Read the model definition and answer for the solid it produces. Units are mm, in the model's axes. Give positions to 0.01 mm unless a question says otherwise; leave off trailing zeros. Order: outer loops, then holes, each group sorted by start corner. A loop starts at its lowest first (then second) coordinate and runs counter-clockwise, first axis right, second up. Notation, with made-up numbers: M 80.25,30.25 L 109.25,30.25 A10 ccw 109.25,38.25 Z; hole C -29,9.5 d11. An arc over 180 degrees is marked long. Write item = value, one per line. Start each with the question number.
from build123d import *

# Parameters (mm, degrees)
SKETCH1_W                    = 25.4
SKETCH1_H                    = 25.4
SKETCH1_W_2                  = 22.225
SKETCH1_H_2                  = 22.225
EXTRUDE_THIN1_DEPTH          = 387.35
F_10_0_1935_DIAMETER_HOLE1_D = 4.9149
F_10_0_1935_DIAMETER_HOLE2_D = 4.9149


with BuildPart() as part:
    # Sketch1 → Extrude-Thin1 (new body)
    with BuildSketch(Plane(origin=(0, 0, 0), x_dir=(0, 0, -1), z_dir=(1, 0, 0))):
        Rectangle(SKETCH1_W, SKETCH1_H)
        Rectangle(SKETCH1_W_2, SKETCH1_H_2, mode=Mode.SUBTRACT)
    extrude(amount=EXTRUDE_THIN1_DEPTH)

    # #10 (0.1935) Diameter Hole1 (through all)
    with Locations(Plane.XY.offset(12.7)):
        with Locations((9.525, 0), (377.825, 0)):
            Hole(F_10_0_1935_DIAMETER_HOLE1_D / 2)

    # #10 (0.1935) Diameter Hole2 (through all)
    with Locations(Plane(origin=(0, 12.7, 0), x_dir=(1, 0, 0), z_dir=(0, 1, 0))):
        with Locations((136.525, -7.9375), (219.075, -7.9375)):
            Hole(F_10_0_1935_DIAMETER_HOLE2_D / 2)


solid = part.part
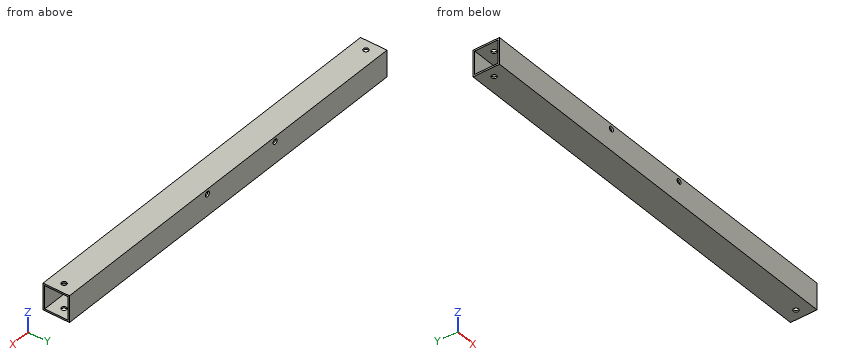
1) Find section B-B on z = -4.25. Determine the outline of the cut face in (x, y).
2) Find the intervals of material crossed by probe 1 along Y at (x, z) = (151, -9.75), in increasing order. Write a range as [from, to].
3) Each of these flat-tipped pins is pushed along its axis until it touches: P1, Ø8, axis at x = 9.525, y = 0, coming from the -Z side; P2, Ø4.5, axis at x = 219.08, z = 7.94, coming from the -Y side. Where does it stop, or does it pass through?
4) Find section A-A on x = 107. Determine the outline of the cut face in (y, z), plus the area to 3 significant figures.
Numbers:
q1.outline = M 0,-12.7 L 387.35,-12.7 L 387.35,-11.11 L 0,-11.11 Z; M 0,11.11 L 387.35,11.11 L 387.35,12.7 L 0,12.7 Z
q2.probe_1 = [-12.7, -11.11], [11.11, 12.7]
q3.P1 = -12.7
q3.P2 = through
q4.outline = M -12.7,-12.7 L 12.7,-12.7 L 12.7,12.7 L -12.7,12.7 Z; hole M -11.11,-11.11 L 11.11,-11.11 L 11.11,11.11 L -11.11,11.11 Z
q4.area = 151 mm2
